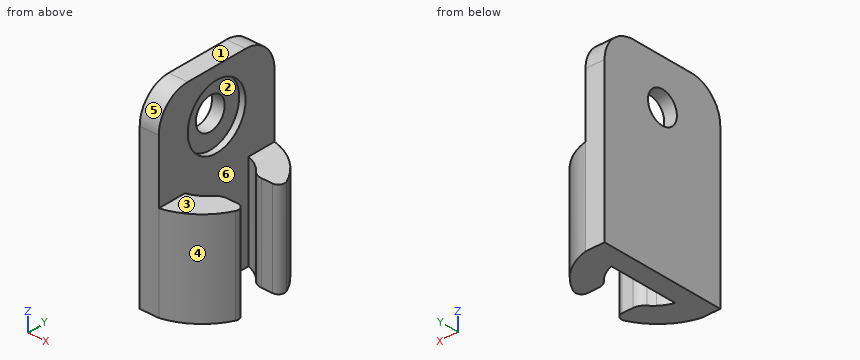
```python
from build123d import *

# Parameters (mm, degrees)
F1_DEPTH = 30
F2_DEPTH = 15
F3_R     = 2.5
F4_DEPTH = 25
F5_R     = 5
F3_R_2   = 5
F6_DEPTH = 1
F7_R     = 2
F8_R     = 1


with BuildPart() as f1:
    # F0 (on Top) → F1 (new body)
    with BuildSketch(Plane.XY):
        Polygon((3, 10), (0, 10), (0, -10), (3, -10), (3, -5.5), (3, 5.5), align=None)
    extrude(amount=F1_DEPTH)

    # F0 (on Top) → F2 (join)
    with BuildSketch(Plane.XY):
        with BuildLine():
            ThreePointArc((10.551148, 3), (7.718324, 7.516978), (3, 10))
            Line((3, 10), (3, 5.5))
            Line((3, 5.5), (5, 5.5))
            Line((5, 5.5), (5, 4.499471))
            ThreePointArc((5, 4.499471), (5.740219, 3.809727), (6.346858, 3))
            Line((6.346858, 3), (10.551148, 3))
        make_face()
        with BuildLine():
            Line((3, -5.5), (3, -10))
            ThreePointArc((3, -10), (7.718324, -7.516978), (10.551148, -3))
            Line((10.551148, -3), (6.346858, -3))
            ThreePointArc((6.346858, -3), (5.740219, -3.809727), (5, -4.499471))
            Line((5, -4.499471), (5, -5.5))
            Line((5, -5.5), (3, -5.5))
        make_face()
        with BuildLine():
            Line((5, 5.5), (3, 5.5))
            ThreePointArc((3, 5.5), (4.049539, 5.09876), (5, 4.499471))
            Line((5, 4.499471), (5, 5.5))
        make_face()
        with BuildLine():
            ThreePointArc((5, -4.499471), (4.049539, -5.09876), (3, -5.5))
            Line((3, -5.5), (5, -5.5))
            Line((5, -5.5), (5, -4.499471))
        make_face()
    extrude(amount=F2_DEPTH)

    # F3 (on face) → F4 (cut)
    with BuildSketch(Plane.YZ.offset(3)):
        with Locations((0, 23)):
            Circle(F3_R)
    extrude(amount=-F4_DEPTH, mode=Mode.SUBTRACT)

    # F5
    f5_edges = [f1.edges().sort_by_distance(p)[0] for p in [
        (1.5, -10, 30),
        (1.5, 10, 30),
    ]]
    fillet(f5_edges, radius=F5_R)

    # F3 (on face) → F6 (cut)
    with BuildSketch(Plane.YZ.offset(3)):
        with Locations((0, 23)):
            Circle(F3_R_2)
        with Locations((0, 23)):
            Circle(F3_R, mode=Mode.SUBTRACT)
    extrude(amount=-F6_DEPTH, mode=Mode.SUBTRACT)

    # F7
    f7_edges = [f1.edges().sort_by_distance(p)[0] for p in [
        (6.346858, -3, 7.5),
        (6.346858, 3, 7.5),
    ]]
    fillet(f7_edges, radius=F7_R)

    # F8
    f8_edges = [f1.edges().sort_by_distance(p)[0] for p in [
        (10.551148, -3, 7.5),
        (10.551148, 3, 7.5),
    ]]
    fillet(f8_edges, radius=F8_R)


solid = f1.part
```
Check sheet for the modelled part. Datum: model origin and axes. Units: mm. Face numbers are marked on the shaded views. A direction names the side the tool comes from. Round coordinates to 2 decimals unless told otherwise and drop trailing zeros. Order: outer loops, then holes, each group sorted by start corner. A loop starts at its lowest first (then second) coordinate and runs counter-clockwise, first axis right, second up. Notation, with made-up numbers: (-32.75, 28.25) -> (13.25, 28.25) arc R22 ccw to (13.25, 46.25) -> close; hole circle Ø10 at (65, 73.5). An arc over 180 degrees is marked (long way). One line per item, written item: value. Start each with the question number.
Q1. Cross-section at D-D (x = 8). Record the boundary of the cut face in (y, z).
Q2. Cross-section at C-C (y = 0). Record the boundary of the cut face in (x, z), and give its area (3 significant figures).
Q3. Cross-section at A-A (x = 1.25). Record the boundary of the cut face in (y, z), and give its area (3 significant figures).
Q4. Gauge pin test, flat ends, axial feed: pin 1 Ø1.9 at (x, z) = (8, 5.5) entering from +Y; pin 2 Ø3 at (y, z) = (1.5, 23.5) entering from +X; pin 3 Ø10 at (y, z) = (3.5, 17) entering from +X; pin 4 Ø1 at (x, z) = (4.5, 14.5) entering from -Y. Record the tip position at first contact, or that the pin passes through.
Q5. Thickness scan on line 1 (Z direction, x = 2.6, y = 0); line 2 (Z direction, x = 1.2, y = 0); line 3 (Z direction, x = 8.5, y = -5.75). Record the ranges inside material, lowest first.
Q6. Mould release check, pull along X, two halves, no side actions. Record for the marked faces 4, 5 and 6: pulls with the +X half, pulls with the -X half, needs draft (parallel to the pull), parting line crosses it, or undercut.
Q7. Set-up check for the marked faces 1, 2 and 3: record each of +Z, -Z, +X, -X, +Y, -Y from which the full face is reachable in a straight line by a thin tool's end or side.
Q8. Cross-section at B-B (z = 23). Record the boundary of the cut face in (x, y).
Completed:
1. outline: (-7.25, 0) -> (-3, 0) -> (-3, 15) -> (-7.25, 15) -> close; (3, 0) -> (7.25, 0) -> (7.25, 15) -> (3, 15) -> close
2. outline: (0, 0) -> (3, 0) -> (3, 18) -> (2, 18) -> (2, 20.5) -> (0, 20.5) -> close; (0, 25.5) -> (2, 25.5) -> (2, 28) -> (3, 28) -> (3, 30) -> (0, 30) -> close
2. area: 70.0 mm²
3. outline: (-10, 0) -> (10, 0) -> (10, 25) arc R5 ccw to (5, 30) -> (-5, 30) arc R5 ccw to (-10, 25) -> close; hole circle Ø5 at (0, 23)
3. area: 570 mm²
4. pin 1: stops at y = 8.09
4. pin 2: stops at x = 2
4. pin 3: stops at x = 10.09
4. pin 4: stops at y = -9.72
5. line 1: z = 0 to 18, 28 to 30
5. line 2: z = 0 to 20.5, 25.5 to 30
5. line 3: z = 0 to 15
6. face 4: pulls with the +X half
6. face 5: needs draft
6. face 6: undercut
7. face 1: +Z, +X, -X, +Y, -Y
7. face 2: +X
7. face 3: +Z, +X, +Y, -Y
8. outline: (0, -10) -> (3, -10) -> (3, -5) -> (2, -5) -> (2, -2.5) -> (0, -2.5) -> close; (0, 2.5) -> (2, 2.5) -> (2, 5) -> (3, 5) -> (3, 10) -> (0, 10) -> close
